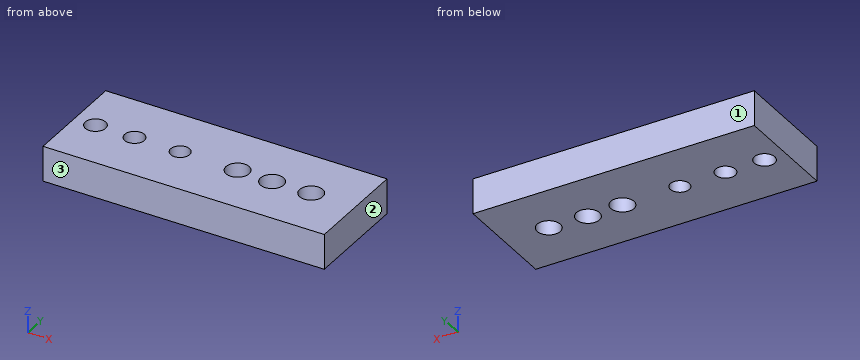
from build123d import *

# Parameters (mm, degrees)
SKETCH_W      = 40
SKETCH_H      = 15
PAD_DEPTH     = 5
SKETCH001_R   = 1.45
SKETCH001_R_2 = 1.4
SKETCH001_R_3 = 1.35
POCKET_DEPTH  = 20
SKETCH002_R   = 1.65
HOLE_DEPTH    = 25


with BuildPart() as part:
    # Sketch → Pad (new body)
    with BuildSketch(Plane.XY):
        Rectangle(SKETCH_W, SKETCH_H)
    extrude(amount=PAD_DEPTH)

    # Sketch001 (on Face6 of Pad) → Pocket (cut)
    with BuildSketch(Plane.XY.offset(5)):
        with Locations((-17, 0)):
            Circle(SKETCH001_R)
        with Locations((-11.444874, 0)):
            Circle(SKETCH001_R_2)
        with Locations((-4.956441, 0)):
            Circle(SKETCH001_R_3)
    extrude(amount=-POCKET_DEPTH, mode=Mode.SUBTRACT)

    # Sketch002 (on Face5 of Pocket) → Hole (cut)
    with BuildSketch(Plane.XY.offset(5)):
        with Locations((3.262239, -0.090117)):
            Circle(SKETCH002_R)
        with Locations((8.236705, -0.198258)):
            Circle(SKETCH002_R)
        with Locations((13.715827, -0.05407)):
            Circle(SKETCH002_R)
    extrude(amount=-HOLE_DEPTH, mode=Mode.SUBTRACT)


solid = part.part
Part model, mm, in its own coordinate system. Face numbers are marked on the shaded views. Coordinates: 2 decimals unless noted, no trailing zeros. Loops run counter-clockwise (first coordinate to the right, second up) from the corner with the lowest first, then second, coordinate; pieces in that order, holes last. Notation, with made-up numbers: (60.25, -31) -> (66.25, -31) arc R16 cw to (66.25, -6) -> close; hole circle Ø3 at (20.5, -1.5). An arc over 180 degrees is marked (long way). Use a Markdown table: item, result. Add a question column.
Item 1: Band-saw the part on C-C on z = 4.15. Write the cut outline in (x, y), plus the area to 3 significant figures.
Item 2: Band-saw the part on B-B on x = -17. Write the cut outline in (y, z).
Item 3: Pull direction Y, two halves, no side cores. Call the marked faces 1, 2 and 3: +Y half, -Y half, draft (parallel to the pull), parting line (faces both ways), or undercut.
Item 4: Probe probe 1 along Y at (x, z) = (-17, 1.65); probe 2 along Y at (x, z) = (4, 1.85). List the from-to ranges inside material, lowest first.
Item 5: Band-saw the part on A-A on y = 0.5. Write the cut outline in (x, z).
Geometry says:
| question | item | result |
|---|---|---|
| 1 | outline | (-20, -7.5) -> (20, -7.5) -> (20, 7.5) -> (-20, 7.5) -> close; hole circle Ø2.9 at (-17, 0); hole circle Ø2.8 at (-11.44, 0); hole circle Ø2.7 at (-4.96, 0); hole circle Ø3.3 at (3.26, -0.09); hole circle Ø3.3 at (8.24, -0.2); hole circle Ø3.3 at (13.72, -0.05) |
| 1 | area | 556 mm² |
| 2 | outline | (-7.5, 0) -> (-1.45, 0) -> (-1.45, 5) -> (-7.5, 5) -> close; (1.45, 0) -> (7.5, 0) -> (7.5, 5) -> (1.45, 5) -> close |
| 3 | face 1 | +Y half |
| 3 | face 2 | draft |
| 3 | face 3 | -Y half |
| 4 | probe 1 | -7.5 to -1.45, 1.45 to 7.5 |
| 4 | probe 2 | -7.5 to -1.57, 1.39 to 7.5 |
| 5 | outline | (-20, 0) -> (-18.36, 0) -> (-18.36, 5) -> (-20, 5) -> close; (-15.64, 0) -> (-12.75, 0) -> (-12.75, 5) -> (-15.64, 5) -> close; (-10.14, 0) -> (-6.21, 0) -> (-6.21, 5) -> (-10.14, 5) -> close; (-3.7, 0) -> (1.72, 0) -> (1.72, 5) -> (-3.7, 5) -> close; (4.8, 0) -> (6.74, 0) -> (6.74, 5) -> (4.8, 5) -> close; (9.73, 0) -> (12.16, 0) -> (12.16, 5) -> (9.73, 5) -> close; (15.27, 0) -> (20, 0) -> (20, 5) -> (15.27, 5) -> close |
